Print and shaded views of the part. All mm, measured from the part's lowest x, y and z. Give positions to 0.01 mm unless a question says otherwise; leave off trailing zeros. Write each loop counter-clockwise with the first axis right and the second up, starting at its lowest first coordinate (ties: lowest second). Pieces come first, ordered by that corner, then holes. Notation, with made-up numbers: M -12.75,47.5 L 11.25,47.5 A12 cw 11.25,56.5 Z; hole C 29.25,24.5 d11. An arc over 180 degrees is marked long. One line per question, with ' | ' between items. Start each with the question number.
1. Cut at B-B, the plane x = 49. Write the cut outline in (y, z).
2. Wall check: L1, parallel to Y at x = 184.5, z = 106.5; L2, parallel to X at y = 513.75, z = 112.5 (1 decimal); L3, parallel to Y at x = 95, z = 261. Give the ranges that are in metal, low to high.
3. Flat gauge pins, fed straight in: pin 1 (7.5 mm diameter, centred on x = 85.05, z = 187.5, fed in from +Y); pin 2 (6 mm diameter, centred on y = 106.5, z = 197.5, fed in from +X); pin 3 (5 mm diameter, centred on x = 164, y = 68.5, fed in from -Z). Where does each tip first touch, or does it go through?
4. Cut at C-C, the plane z = 277. Write the cut outline in (x, y), then the cut area to 3 significant figures.
5. Cut at A-A, the plane y = 173.5. Write the cut outline in (x, z), then the cut area to 3 significant figures.
6. Pull direction Y, two halves, no side cores. Call the marked faces 1, 2 and 3: released by +Y, released by -Y, zero draft, split by the parting line, or undercut.
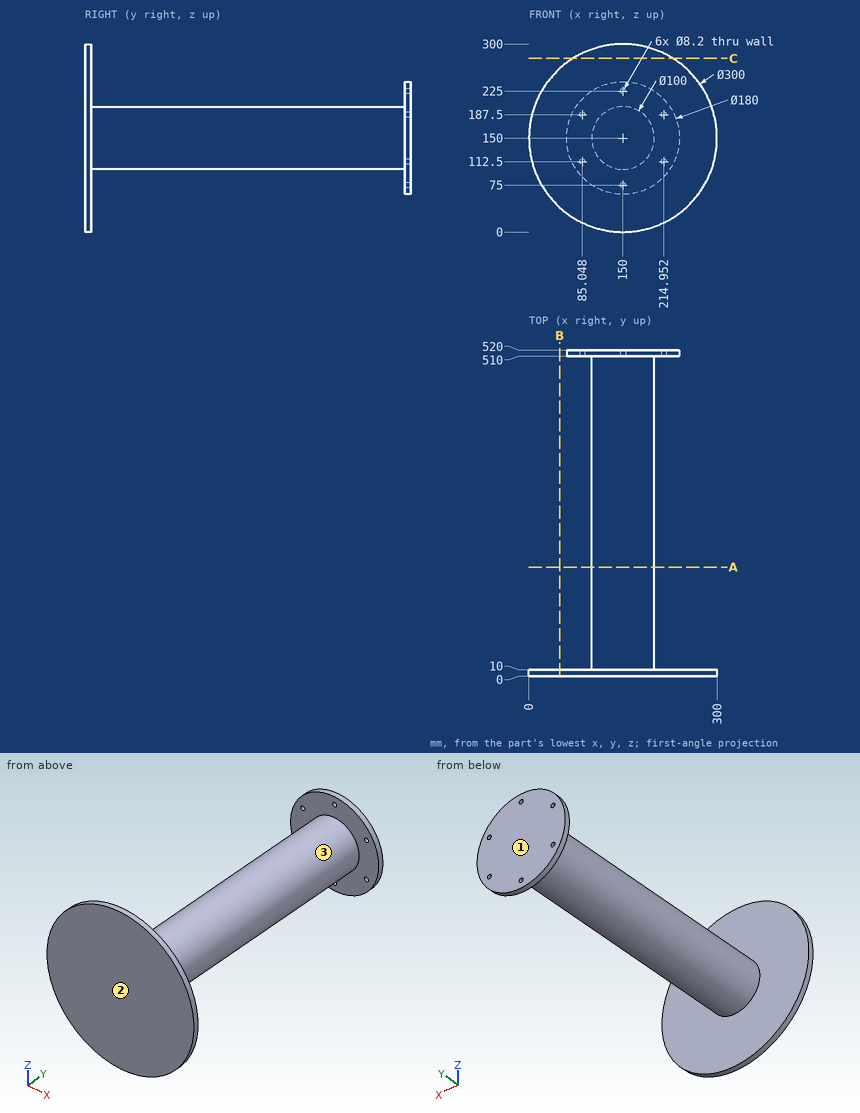
Here are the results:
1) outline: M 0,39.1 L 10,39.1 L 10,260.9 L 0,260.9 Z
2) L1: 0 to 10, 510 to 520 | L2: 68.2 to 80.9, 89.1 to 210.9, 219.1 to 231.8 | L3: 0 to 10
3) pin 1: y = 10 | pin 2: x = 172.8 | pin 3: z = 101.34
4) outline: M 70.18,0 L 229.82,0 L 229.82,10 L 70.18,10 Z | area: 1,600 mm^2
5) outline: C 150,150 d100 | area: 7,850 mm^2
6) face 1: released by +Y | face 2: released by -Y | face 3: undercut
